Part model, mm, in its own coordinate system. A direction names the side the tool comes from. Round coordinates to 2 decimals unless told otherwise and drop trailing zeros. Write each loop counter-clockwise with the first axis right and the second up, starting at its lowest first coordinate (ties: lowest second). Pieces come first, ordered by that corner, then holes. Notation, with made-up numbers: M 29,-28 L 52,-28 A24 cw 52,-8 Z; hole C 56,-5 d9. An arc over 180 degrees is marked long. Answer as a JSON object with one key per item and string values. Group by question number.
1. Band-saw the part on C-C, the plane z = 6. Write the cut outline in (x, y).
2. Band-saw the part on A-A, the plane x = 26.5. Write the cut outline in (y, z), plus the area to 3 significant figures.
3. Drill centre lines: line 1 (X direction, y = -2, z = 15.5); line 2 (Y direction, x = -3, z = 20); line 3 (Z direction, x = -35, y = 23.5). Where is each one in solid material? Low to high. Write a range as from..to.
4. Drop flat-ended pins along their axis: pin 1 (3 mm diameter, centred on y = 19, z = 32, fed in from -X); pin 2 (8 mm diameter, centred on x = -6.5, y = 25, fed in from +Z). Give the stop position or say it passes through.
5. Which spindle directions (+Z, -Z, +X, -X, +Y, -Y) get a long thin tool onto all of the face, cutting with end or side? Do faces 5 (the face through (-27.43, 25.13, 37.92)), 6 (the face through (-45.727, -1, 13)). Say none if no direction does.
6. Band-saw the part on D-D, the plane y = -38.5. Write the cut outline in (x, z), plus the area to 3 significant figures.
7. Band-saw the part on B-B, the plane y = -14. Write the cut outline in (x, z), plus the area to 3 significant figures.
8. Two-plate mould, pull along X, no slides. Class faces 1 (the face through (13.15, -3.73, 12.88)), 2 (the face through (-1, 51.952, 13)), 3 (the face through (30.787, -4, 13)), 4 (the face through (45.727, -1, 13)): +X half, -X half, draft (parallel to the pull), parting line (faces both ways), or undercut.
from build123d import *

# Parameters (mm, degrees)
F0_W     = 91.4542
F0_H     = 103.904634
F1_DEPTH = 25.4
F2_R     = 7.743106
F3_DEPTH = 25.4
F4_DEPTH = 25.4


with BuildPart() as f1:
    # F0 (on Top) → F1 (new body)
    with BuildSketch(Plane.XY):
        Rectangle(F0_W, F0_H)
    extrude(amount=F1_DEPTH)

    # F2 (on face) → F3 (join)
    with BuildSketch(Plane.XY.offset(25.4)):
        with Locations((-19.694343, 24.787709)):
            Circle(F2_R)
    extrude(amount=F3_DEPTH)

    # F2 (on face) → F4 (cut)
    with BuildSketch(Plane.XY.offset(25.4)):
        Polygon((30.786563, 20.713016), (-4.980177, -28.8624), (30.786563, -27.956914), align=None)
    extrude(amount=-F4_DEPTH, mode=Mode.SUBTRACT)


solid = f1.part
Worked answers:
{
 "1": {"outline": "M -45.73,-51.95 L 45.73,-51.95 L 45.73,51.95 L -45.73,51.95 Z; hole M -4.98,-28.86 L 30.79,-27.96 L 30.79,20.71 Z"},
 "2": {"outline": "M -51.95,0 L -28.07,0 L -28.07,25.4 L -51.95,25.4 Z; M 14.77,0 L 51.95,0 L 51.95,25.4 L 14.77,25.4 Z", "area": "1,550 mm^2"},
 "3": {"line 1": "x = -45.73..14.4, 30.79..45.73", "line 2": "y = -51.95..-28.81, -26.12..51.95", "line 3": "z = 0..25.4"},
 "4": {"pin 1": "stops at x = -26.14", "pin 2": "stops at z = 25.4"},
 "5": {"face 5": "+Z", "face 6": "+Z, -Z, -X, +Y, -Y"},
 "6": {"outline": "M -45.73,0 L 45.73,0 L 45.73,25.4 L -45.73,25.4 Z", "area": "2,320 mm^2"},
 "7": {"outline": "M -45.73,0 L 5.74,0 L 5.74,25.4 L -45.73,25.4 Z; M 30.79,0 L 45.73,0 L 45.73,25.4 L 30.79,25.4 Z", "area": "1,690 mm^2"},
 "8": {"face 1": "undercut", "face 2": "draft", "face 3": "undercut", "face 4": "+X half"}
}
